```python
from build123d import *

# Parameters (mm, degrees)
BOSS_EXTRUDE1_DEPTH = 2


with BuildPart() as part:
    # Sketch2 → Boss-Extrude1 (new body)
    with BuildSketch(Plane(origin=(0, 0, 0), x_dir=(1, 0, 0), z_dir=(0, 1, 0))):
        with BuildLine():
            Line((377.810759056, 1640.360670751), (377.762780786, 1638.727684223))
            Line((377.762780786, 1638.727684223), (377.762780786, 1637.032768164))
            ThreePointArc((377.762780786, 1637.032768164), (377.973133338, 1636.52493218), (378.480969321, 1636.314579628))
            Line((378.480969321, 1636.314579628), (381.034322317, 1636.314579628))
            Line((381.034322317, 1636.314579628), (383.53259373, 1637.921344077))
            Line((383.53259373, 1637.921344077), (383.53259373, 1648.93129383))
            Line((383.53259373, 1648.93129383), (382.997065463, 1649.428721271))
            Line((382.997065463, 1649.428721271), (378.071384282, 1649.428721271))
            ThreePointArc((378.071384282, 1649.428721271), (376.912121238, 1650.587984315), (378.071384282, 1651.747247359))
            Line((378.071384282, 1651.747247359), (385.733950351, 1651.747247359))
            Line((385.733950351, 1651.747247359), (386.145150231, 1652.107387132))
            Line((386.145150231, 1652.107387132), (385.251957701, 1722.695235293))
            ThreePointArc((385.251957701, 1722.695235293), (385.107061178, 1723.280508889), (384.717360317, 1723.740588689))
            Line((384.717360317, 1723.740588689), (377.294522639, 1723.740588689))
            ThreePointArc((377.294522639, 1723.740588689), (376.703471551, 1724.331639778), (377.294522639, 1724.922690866))
            Line((377.294522639, 1724.922690866), (383.5733207, 1724.922690866))
            Line((383.5733207, 1724.922690866), (384.893964101, 1725.772063299))
            Line((384.893964101, 1725.772063299), (384.893964101, 1735.694301181))
            ThreePointArc((384.893964101, 1735.694301181), (384.606449822, 1736.388422052), (383.912328951, 1736.675936331))
            Line((383.912328951, 1736.675936331), (373.489641238, 1736.675936331))
            ThreePointArc((373.489641238, 1736.675936331), (372.1028909, 1738.062686668), (373.489641238, 1739.449437006))
            Line((373.489641238, 1739.449437006), (379.048025738, 1739.449437006))
            Line((379.048025738, 1739.449437006), (380.205497535, 1740.065323077))
            Line((380.205497535, 1740.065323077), (380.205497535, 1748.201358299))
            Line((380.205497535, 1748.201358299), (371.764667819, 1748.201358299))
            Line((371.764667819, 1748.201358299), (371.408873695, 1764.738317132))
            ThreePointArc((371.408873695, 1764.738317132), (371.619067882, 1765.278343177), (372.149553695, 1765.511569521))
            Line((372.149553695, 1765.511569521), (377.810759056, 1765.511569521))
            ThreePointArc((377.810759056, 1765.511569521), (379.185604537, 1766.148142401), (379.589611464, 1767.608349076))
            Line((379.589611464, 1767.608349076), (379.589611464, 1781.024075112))
            Line((379.589611464, 1781.024075112), (271.404811714, 1779.291132304))
            Line((271.404811714, 1779.291132304), (267.990517204, 1778.686872698))
            Line((267.990517204, 1778.686872698), (264.479907812, 1774.907365565))
            Line((264.479907812, 1774.907365565), (268.781456477, 1574.975639595))
            Line((268.781456477, 1574.975639595), (272.687420737, 1570.633405031))
            Line((272.687420737, 1570.633405031), (373.489641238, 1570.633405031))
            Line((373.489641238, 1570.633405031), (374.425169749, 1571.4749397))
            Line((374.425169749, 1571.4749397), (373.553861857, 1640.333273274))
            ThreePointArc((373.553861857, 1640.333273274), (375.668526286, 1642.488694532), (377.810759056, 1640.360670751))
        make_face()
    extrude(amount=BOSS_EXTRUDE1_DEPTH)


solid = part.part
```
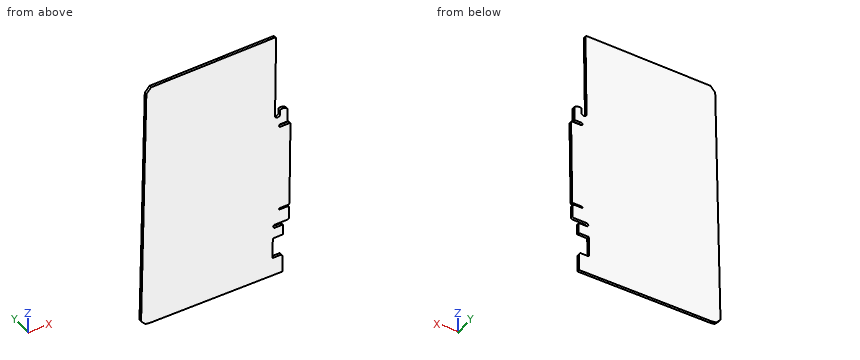
The model under review builds one solid part; all positions refer to its coordinate system, in mm. Round coordinates to 2 decimals unless told otherwise and drop trailing zeros. Order: outer loops, then holes, each group sorted by start corner. A loop starts at its lowest first (then second) coordinate and runs counter-clockwise, first axis right, second up.
Item 1: To check wall thickness, follow probe 1 along Z at (x, y) = (380.5, 0.6); probe 2 along Z at (x, y) = (381.5, 1.55); probe 3 along X at (y, z) = (0.2, -1641). State the ranges of each line that lie inside material, in increasing order.
Working result:
probe 1: z = -1736.68 to -1724.92, -1723.74 to -1651.75, -1649.43 to -1636.31
probe 2: z = -1736.68 to -1724.92, -1723.74 to -1651.75, -1649.43 to -1636.61
probe 3: x = 267.36 to 373.65, 377.71 to 383.53
Item 2: Add section A-A, the plane z = -1682. State the section outline as (x, y) points.
Working result:
outline: (266.48, 0) - (385.77, 0) - (385.77, 2) - (266.48, 2) - close
Item 3: For pin 1 (1 mm diameter, centred on x = 379.5, y = 1, fed in from +Z); pin 2 (1 mm diameter, centred on x = 343, y = 0.5, fed in from -Z); pin 3 (1 mm diameter, centred on x = 375, y = 0.5, fed in from +Z), all flat-tipped, find the tip position at first contact; note any pin that passes through.
Working result:
pin 1: stops at z = -1636.31
pin 2: stops at z = -1780.45
pin 3: stops at z = -1642.13
